Geometry: final body of the model. Coordinates: model frame, mm. Face numbers are marked on the shaded views. A direction names the side the tool comes from. Coordinates: 2 decimals unless noted, no trailing zeros. Order: outer loops, then holes, each group sorted by start corner. A loop starts at its lowest first (then second) coordinate and runs counter-clockwise, first axis right, second up. Notation, with made-up numbers: M 16.25,39 L 53.25,39 A34 ccw 53.25,78 Z; hole C 80,33.25 d7. An arc over 180 degrees is marked long. Use CSV: the item, a comma, the result in double quotes. Start each with the question number.
Q1. First-contact query: P1, Ø8, axis at y = 51, z = 26, coming from the +X side; P2, Ø3, axis at y = -13.5, z = 15.5, coming from the -X side; P3, Ø6, axis at x = -12.5, y = 39.5, coming from the -Z side. Flat tips, straight axial feed; report the tip coordinate or a pass-through.
Q2. Section query B-B, the plane y = -8.5. Output: boundary loops of the cut face in (x, z).
Q3. Access query for the marked faces 1 and 2. Directions: +Z, -Z, +X, -X, +Y, -Y. A direction counts if a zero-diameter tool reaches every point of the face in a straight line with its end or side. Return the directions, or none.
Q4. Section query A-A, the plane z = 26.5. Output: boundary loops of the cut face in (x, y), and give its area (3 significant figures).
Q5. Ray query, probe 1 along X at (y, z) = (18.5, 19.5); probe 2 along Y at (x, z) = (-27, 41.5); probe 3 along Y at (x, z) = (-9.5, 59.5). Return the intervals inside material, ascending.
Q6. Section query D-D, the plane z = 7. Output: boundary loops of the cut face in (x, y), and give its area (3 significant figures).
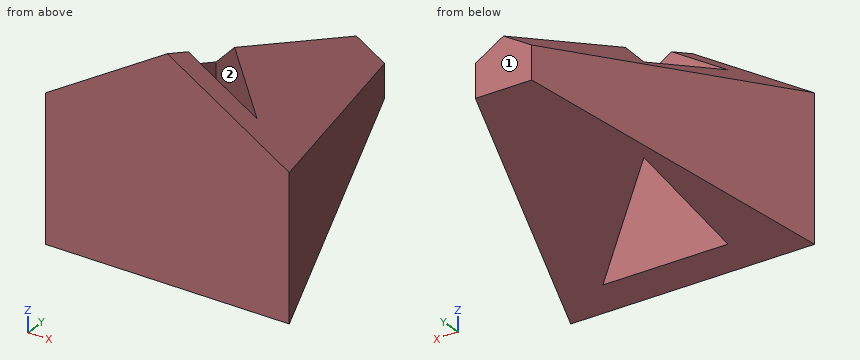
Autodesk Inventor part; units mm, degrees
ref_plane "РабПлоскость1" through (-53.4198, -27.106, 46) normal (-0.4959, 0.3237, 0.8058) x (0.8517, 0, 0.5241)
ref_plane "РабПлоскость2" through (24.5802, -27.106, 46) normal (-0.4959, -0.3237, -0.8058) x (-0.8517, 0, 0.5241)
ref_plane "РабПлоскость3" through (24.5802, -27.106, 0) normal (-0.9487, -0.3162, 0) x (0, 0, 1)
sketch "Эскиз1" plane through (0, 0, 0) normal (0, 0, 1) x (1, 0, 0)
  line L0 (-53.4198, 62.894) -> (24.5802, 62.894)
  line L1 (24.5802, 62.894) -> (24.5802, -27.106)
  line L2 (24.5802, -27.106) -> (-53.4198, -27.106)
  line L3 (-53.4198, -27.106) -> (-53.4198, 62.894)
  line L4 (7.5802, -17.106) -> (-32.4198, -17.106)
  line L5 (-32.4198, -17.106) -> (-32.4198, 22.894)
  line L6 (-32.4198, 22.894) -> (7.5802, -17.106)
  point P0 (0, 0)
  point P1 (-14.4198, -27.106)
  point P2 (-14.4198, -17.106)
  dimension "d0" = 78
  dimension "d1" = 90
  dimension "d4" = 18
  dimension "d5" = 0
  dimension "d6" = 40
  dimension "d7" = 40
  dimension "d8" = 10
extrude "Выдавливание1" add sketch "Эскиз1" along normal blind 70
sketch "Эскиз3" plane through (-53.4198, 62.894, 0) normal (0, 1, 0) x (1, 0, 0)
  line L0 (78, -70) -> (0, -70)
  line L1 (39, -70) -> (78, -46)
  line L2 (78, 0) -> (78, -70)
  line L3 (78, 0) -> (0, 0)
  line L4 (39, -70) -> (0, -46)
  line L5 (0, 0) -> (0, -70)
  line L6 (0, -46) -> (0, 0)
  line L7 (0, 0) -> (78, 0)
  line L8 (78, 0) -> (78, -46)
  point P0 (53.4198, 0)
  dimension "d14" = 46
extrude "Выдавливание2" cut sketch "Эскиз3" against normal blind 1000 contours L4 L5 L3 L2 L1 keep common part
sketch "Эскиз4" plane through (-53.4198, 62.894, 0) normal (0, 1, 0) x (1, 0, 0)
  line L0 (78, 0) -> (0, 0)
  line L1 (0, 0) -> (78, 0)
  line L2 (0, 0) -> (0, -46)
  line L3 (0, -23) -> (78, -23)
  line L4 (78, 0) -> (78, -46)
  line L5 (39, -23) -> (78, 0)
  line L6 (78, -46) -> (39, -70)
  line L7 (39, -23) -> (78, -46)
  line L8 (39, -23) -> (0, -46)
  line L9 (39, -23) -> (0, 0)
  line L10 (30, -17.6923) -> (48, -17.6923)
  line L11 (48, -17.6923) -> (48, -28.3077)
  line L12 (48, -28.3077) -> (30, -28.3077)
  line L13 (30, -28.3077) -> (30, -17.6923)
  line L14 (39, -70) -> (61, -56.4615)
  line L15 (39, -23) -> (39, -70)
  line L16 (48, -28.3077) -> (39, -33.8468)
  line L17 (39, -33.8468) -> (30, -28.3077)
  point P0 (53.4198, 0)
  point P1 (39, -17.6923)
  point P2 (30, -23)
  dimension "d17" = 23
  dimension "d18" = 18
  dimension "d19" = 0
  dimension "d20" = 62.137
  dimension "d21" = 0
  dimension "d22" = 62.14
ref_plane "РабПлоскость1" through (-53.4198, -27.106, 46) normal (-0.4959, 0.3237, 0.8058) x (0.8517, 0, 0.5241)
ref_plane "РабПлоскость2" through (24.5802, -27.106, 46) normal (-0.4959, -0.3237, -0.8058) x (-0.8517, 0, 0.5241)
ref_plane "РабПлоскость3" through (24.5802, -27.106, 0) normal (-0.9487, -0.3162, 0) x (0, 0, 1)
ref_plane "РабПлоскость4" through (-53.4198, -27.106, 0) normal (0, -0.1929, 0.9812) x (1, 0, 0)
ref_plane "РабПлоскость5" through (-53.4198, -27.106, 46) normal (0.9487, -0.3162, 0) x (0, 0, -1)
sketch "Эскиз5" plane through (24.5802, -27.106, 46) normal (-0.4959, -0.3237, -0.8058) x (-0.8517, 0, 0.5241)
  circle A0 centre (16.0933, 68.0296) radius 120.9619
  point P0 (-3.1746, 42.498)
extrude "Выдавливание3" cut sketch "Эскиз5" along normal blind 1000 keep common part
sketch "Эскиз6" plane through (-53.4198, -27.106, 46) normal (-0.4959, 0.3237, 0.8058) x (0.8517, 0, 0.5241)
  circle A0 centre (5.8398, 44.8642) radius 111.1599
  point P0 (21.3869, 47.3906)
extrude "Выдавливание4" cut sketch "Эскиз6" against normal blind 1000 keep common part
sketch "Эскиз7" plane through (24.5802, -27.106, 0) normal (-0.9487, -0.3162, 0) x (0, 0, 1)
  circle A0 centre (24.0277, 56.8574) radius 86.5432
  point P0 (0, 33.4879)
extrude "Выдавливание5" cut sketch "Эскиз7" along normal blind 1000 keep common part
sketch "Эскиз8" plane through (-53.4198, -27.106, 0) normal (0, -0.1929, 0.9812) x (1, 0, 0)
  circle A0 centre (24.124, 48.0247) radius 96.9769
  point P0 (53.4198, 26.5969)
extrude "Выдавливание6" cut sketch "Эскиз8" along normal blind 1000 keep common part
sketch "Эскиз9" plane through (-53.4198, -27.106, 46) normal (0.9487, -0.3162, 0) x (0, 0, -1)
  circle A0 centre (10.0162, 69.3054) radius 109.293
  point P0 (46, 42.6078)
extrude "Выдавливание7" cut sketch "Эскиз9" along normal blind 1000 keep common part
properties part number "1_1"
Responses:
1,P1,"stops at x = -0.12"
1,P2,"stops at x = -49.38"
1,P3,"stops at z = 12.5"
2,outline,"M -47.22,3.66 L -32.42,3.66 L -32.42,51.45 L -47.22,42.34 Z; M -1.03,3.66 L 18.38,3.66 L 18.38,42.34 L -1.03,54.28 Z"
3,face 1,"+Z, -Z, +X, -X, +Y"
3,face 2,"+Z, -Z"
4,outline,"M -53.42,-27.11 L 24.58,-27.11 L -5.42,62.89 L -23.42,62.89 Z; hole M -32.42,-17.11 L 7.58,-17.11 L -32.42,22.89 Z"
4,area,"3,520 mm²"
5,probe 1,"x = -38.22 to -32.42, -28.03 to 9.38"
5,probe 2,"y = -27.11 to -17.11, 17.47 to 24.57"
5,probe 3,"y = -27.11 to -17.11"
6,outline,"M -53.42,-27.11 L 24.58,-27.11 L 12.71,8.5 L -18.03,8.5 L 7.58,-17.11 L -32.42,-17.11 L -32.42,8.5 L -41.55,8.5 Z"
6,area,"1,660 mm²"
